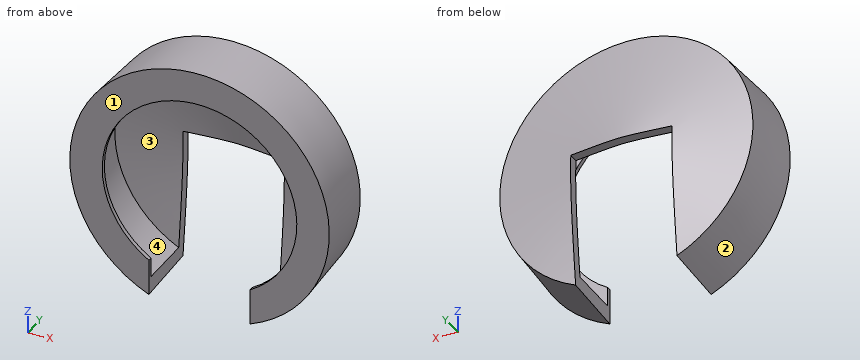
Autodesk Inventor part; units mm, degrees
ref_plane "YZ Plane" through (0, 0, 0) normal (1, 0, 0) x (0, 1, 0)
ref_plane "XZ Plane" through (0, 0, 0) normal (0, 1, 0) x (-1, 0, 0)
ref_plane "XY Plane" through (0, 0, 0) normal (0, 0, 1) x (1, 0, 0)
sketch "Sketch1" plane through (0, 0, 0) normal (1, 0, 0) x (0, 1, 0)
  line L0 (74.9127, 161.4228) -> (59.7618, 161.4228)
  line L1 (-45.1093, -18.0862) -> (-45.1093, 9.0228)
  line L2 (-45.1093, 9.0228) -> (-51.4593, 9.0228)
  line L3 (-51.4593, 9.0228) -> (-51.4593, -41.7772)
  line L4 (37.2342, -18.0862) -> (-45.1093, -18.0862)
  line L5 (-51.4593, -41.7772) -> (50.0237, -36.9026)
  line L6 (50.0237, -36.9026) -> (74.9127, 161.4228)
  line L7 (59.7618, 161.4228) -> (37.2342, -18.0862)
  point P0 (0, 0)
  dimension "d0" = 101.6
  dimension "d2" = 50.8
  dimension "d3" = 6.35
  dimension "d4" = 87.25
revolve "Revolution1" add sketch "Sketch1" angle 360 about axis through (0, 74.9127, 161.4228) along (0, -1, 0)
sketch "Sketch2" plane through (0, -51.4593, 161.4228) normal (0, -1, 0) x (1, 0, 0)
  line L0 (79.375, 25.4) -> (-79.375, 25.4)
  line L1 (-79.375, 25.4) -> (-79.375, -278.9965)
  line L2 (-79.375, -278.9965) -> (79.375, -278.9965)
  line L3 (79.375, -278.9965) -> (79.375, 25.4)
  circle A0 centre (0, 0) radius 203.2
  point P0 (0, -161.4228)
  dimension "d6" = 158.75
  dimension "d7" = 79.375
  dimension "d8" = 25.4
extrude "Extrusion1" cut sketch "Sketch2" against normal blind 127 contours L3 A0 L1 L0 | L3 L2 L1 A0 picked at (-3.0192, -50.7327)
properties part number "FullTopx"
Design review of the part built by this model. Coordinates are the model's own, in mm. Face numbers are marked on the shaded views. Give positions to 0.01 mm unless a question says otherwise; leave off trailing zeros. Loops run counter-clockwise (first coordinate to the right, second up) from the corner with the lowest first, then second, coordinate; pieces in that order, holes last. Notation, with made-up numbers: M 89,-22 L 141,-22 A30 ccw 141,2 Z; hole C -25,28.25 d6. An arc over 180 degrees is marked long. Write item = value, one per line.
Q1. We need section B-B (y = -16). Give the boundary of the cut face in (x, z) (3 decimals).
Output values:
outline = M -79.375,-23.781 L -79.375,0.416 A179.509 cw long 79.375,0.416 L 79.375,-23.781 A201.497 ccw long Z
Q2. We need section A-A (x = 0). Give the boundary of the cut face in (y, z), plus the area to 3 significant figures.
Output values:
outline = M -51.46,313.82 L -45.11,313.82 L -45.11,340.93 L 37.23,340.93 L 56.57,186.82 L 71.73,186.82 L 50.02,359.75 L -51.46,364.62 Z
area = 4,690 mm^2
Q3. To check wall thickness, follow line 1 (Y direction, x = -148.5, z = 98); line 2 (X direction, y = 13, z = 326.5); line 3 (Z direction, x = 107.5, y = 5). State the ranges of each line that lie inside material, in increasing order. Write a range as [from, to].
Output values:
line_1 = [-51.46, -45.11], [39.5, 54.65]
line_2 = [-113.1, -70.52], [70.52, 113.1]
line_3 = [-7.81, 17.66], [305.18, 330.65]
Q4. We need section C-C (y = 31). Give the boundary of the cut face in (x, z) (3 decimals).
Output values:
outline = M -79.375,-21.323 L -79.375,0.416 A179.509 cw long 79.375,0.416 L 79.375,-21.323 A199.239 ccw long Z
Q5. Draft analysis for pull direction Y (two halves, no side actions). For the marked faces 1, 2, 3 and 4, state which applies: +Y half, -Y half, draft (parallel to the pull), parting line (faces both ways), or undercut.
Output values:
face_1 = -Y half
face_2 = +Y half
face_3 = undercut
face_4 = undercut
Q6. Insertion check: pin 1 (4 mm diameter, centred on x = -62, y = 0.5, fed in from -Z); pin 2 (10 mm diameter, centred on x = 73.5, z = 288, fed in from +Y); pin 3 (18 mm diameter, centred on x = -30.5, y = 60, fed in from -Z). Each pin has a flat end and moves straight along its axis. Give the tip position at first contact, or say it passes through.
Output values:
pin_1 = 329.14
pin_2 = 57.17
pin_3 = 186.82
